Verification items for this drawing (mm, ordinates from the low corner). A direction names the side the tool comes from. Give positions to 0.01 mm unless a question says otherwise; leave off trailing zeros. Write each loop counter-clockwise with the first axis right and the second up, starting at its lowest first coordinate (ties: lowest second). Pieces come first, ordered by that corner, then holes. Notation, with made-up numbers: M 79,-40 L 110,-40 A23 ccw 110,-29 Z; hole C 78.5,25 d3. An arc over 180 degrees is marked long. Write each question's results on one line, items separated by ' | '.
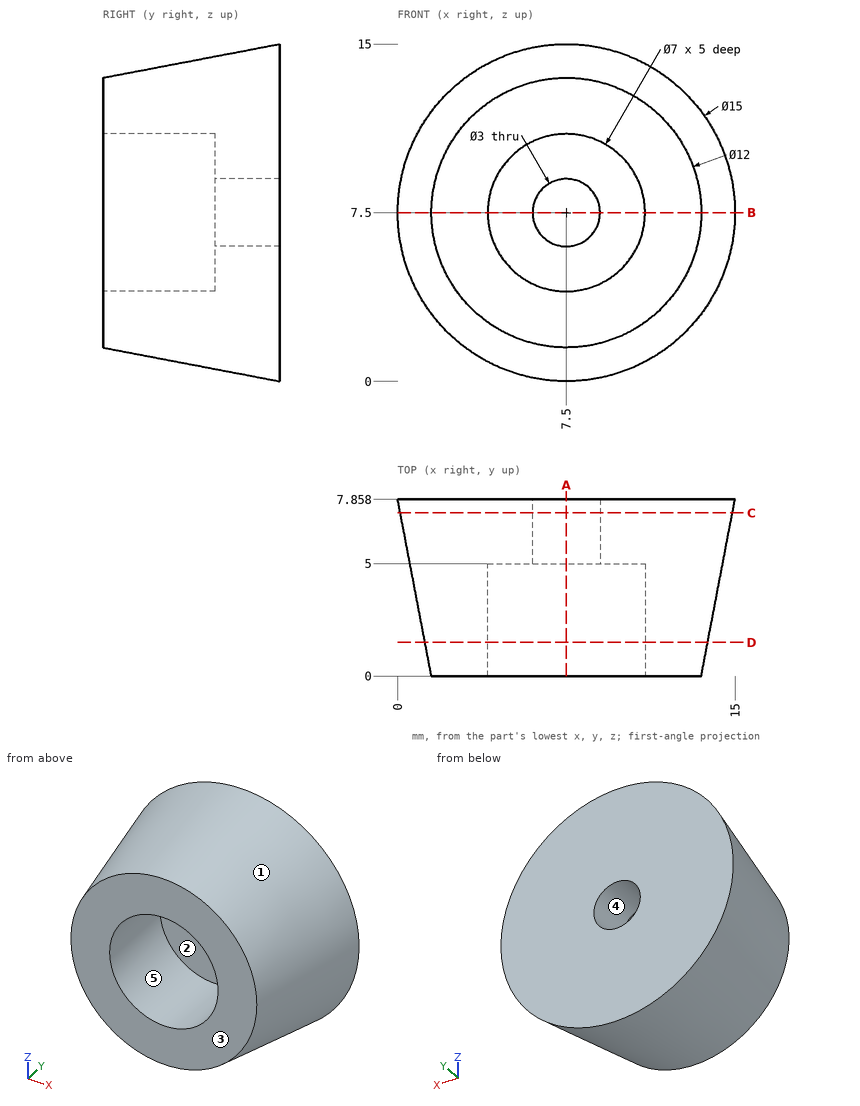
Q1. Section check B-B (z = 7.5). Enter the section's corners in (x, y).
Answer key:
outline: M 0,7.86 L 1.5,0 L 4,0 L 4,5 L 6,5 L 6,7.86 Z; M 9,5 L 11,5 L 11,0 L 13.5,0 L 15,7.86 L 9,7.86 Z
Q2. Section check A-A (x = 7.5). Enter the section's corners in (y, z).
Answer key:
outline: M 0,1.5 L 7.86,0 L 7.86,6 L 5,6 L 5,4 L 0,4 Z; M 0,11 L 5,11 L 5,9 L 7.86,9 L 7.86,15 L 0,13.5 Z
Q3. Access from +Z, -Z, +X, -X, +Y, -Y to the whole of each face (thin tool, end or side, straight path). Record for the marked faces 4 and 5.
Answer key:
face 4: +Y, -Y | face 5: -Y
Q4. Release check for a two-part mould opening along X. For the marked faces 1, 2 and 3 record: released by +X, released by -X, zero draft, split by the parting line, or undercut.
Answer key:
face 1: split by the parting line | face 2: undercut | face 3: zero draft
Q5. Depth check by flat-ended pin: P1, Ø7.5, axis at x = 8, z = 8, coming from the -Y side; P2, Ø2, axis at x = 12, y = 7, coming from the -Z side; P3, Ø1.5, axis at x = 8, y = 1.5, coming from the +Z side; P4, Ø2.5, axis at x = 7.5, z = 7.5, coming from the +Y side. Enter the tip coordinate at first touch or a pass-through.
Answer key:
P1: stops at y = 0 | P2: stops at z = 1.01 | P3: stops at z = 13.92 | P4: passes through
Q6. Section check D-D (y = 1.5). Enter the section's corners in (x, z).
Answer key:
outline: C 7.5,7.5 d12.57; hole C 7.5,7.5 d7
Q7. Section check C-C (y = 7.25). Enter the section's corners in (x, z), then the cut area to 3 significant figures.
Answer key:
outline: C 7.5,7.5 d14.77; hole C 7.5,7.5 d3 | area: 164 mm2
Q8. Material ranges on probe 1 along X at (y, z) = (3, 5.5); probe 2 along Z at (x, y) = (7.5, 1.85); probe 3 along X at (y, z) = (3.8, 7.5), recorded low to high. Write a range as [from, to].
Answer key:
probe 1: x = [1.24, 4.63], [10.37, 13.76] | probe 2: z = [1.15, 4], [11, 13.85] | probe 3: x = [0.77, 4], [11, 14.23]
